```python
from build123d import *

# Parameters (mm, degrees)
BOSS_EXTRUDE1_DEPTH = 3
BOSS_EXTRUDE2_DEPTH = 3
CUT_EXTRUDE1_DEPTH  = 406.369387103
FILLET1_R           = 5
FILLET2_R           = 3.5


with BuildPart() as part:
    # Sketch1 → Boss-Extrude1 (new, symmetric)
    with BuildSketch(Plane(origin=(0, 0, 0), x_dir=(1, 0, 0), z_dir=(0, 1, 0))):
        with BuildLine():
            Line((397, -7.7), (-397, -7.7))
            ThreePointArc((-397, -7.7), (-404.7, 0), (-397, 7.7))
            Line((-397, 7.7), (397, 7.7))
            ThreePointArc((397, 7.7), (404.7, 0), (397, -7.7))
        make_face()
        with BuildLine():
            Line((397, -6.2), (-397, -6.2))
            ThreePointArc((-397, -6.2), (-403.2, 0), (-397, 6.2))
            Line((-397, 6.2), (397, 6.2))
            ThreePointArc((397, 6.2), (403.2, 0), (397, -6.2))
        make_face(mode=Mode.SUBTRACT)
    extrude(amount=BOSS_EXTRUDE1_DEPTH, both=True)

    # Sketch2 → Boss-Extrude2 (add, symmetric)
    with BuildSketch(Plane(origin=(0, 0, 0), x_dir=(1, 0, 0), z_dir=(0, 1, 0))):
        Polygon((-36.145786863, -11.5), (-36.145786863, -14.5), (-36.145786863, -22.5), (-37.645786863, -22.5), (-37.645786863, -12.137653431), (-43.807502688, -6.2), (-41.645786863, -6.2), align=None)
        Polygon((14.854213137, -14.5), (14.854213137, -11.5), (20.354213137, -6.2), (22.515928962, -6.2), (16.354213137, -12.137653431), (16.354213137, -22.5), (14.854213137, -22.5), align=None)
    extrude(amount=BOSS_EXTRUDE2_DEPTH, both=True)

    # Sketch3 → Cut-Extrude1 (cut, through all)
    with BuildSketch(Plane(origin=(0, 3, 0), x_dir=(1, 0, 0), z_dir=(0, 1, 0))):
        Polygon((-40.089183089, -7.7), (-41.645786863, -6.2), (20.354213137, -6.2), (18.797609364, -7.7), align=None)
    extrude(amount=-CUT_EXTRUDE1_DEPTH, mode=Mode.SUBTRACT)

    # Fillet1
    fillet1_edges = [part.edges().sort_by_distance(p)[0] for p in [
        (-36.145786863, 0, 11.5),
        (14.854213137, 0, 11.5),
        (-41.645786863, 0, 6.2),
        (20.354213137, 0, 6.2),
    ]]
    fillet(fillet1_edges, radius=FILLET1_R)

    # Fillet2
    fillet2_edges = [part.edges().sort_by_distance(p)[0] for p in [
        (-42.250898914, 0, 7.7),
        (-37.645786863, 0, 12.137653431),
        (20.959325189, 0, 7.7),
        (16.354213137, 0, 12.137653431),
    ]]
    fillet(fillet2_edges, radius=FILLET2_R)


solid = part.part
```
Verification items for the finished model (mm, model axes). Round coordinates to 2 decimals unless told otherwise and drop trailing zeros. Write each loop counter-clockwise with the first axis right and the second up, starting at its lowest first coordinate (ties: lowest second). Pieces come first, ordered by that corner, then holes.
1. Section check B-B on x = -107. Enter the section's corners in (y, z), plus the area to 3 significant figures.
2. Gauge pin test, flat ends, axial feed: P1, Ø1.8, axis at y = 0.5, z = 19.5, coming from the +X side; P2, Ø1, axis at y = -0.5, z = 0.5, coming from the -X side; P3, Ø1.8, axis at x = 94, y = 1.5, coming from the +Z side; P4, Ø3, axis at y = 0, z = 17, coming from the -X side. Record the tip position at first contact, or that the pin passes through.
3. Section check C-C on y = 0.5. Enter the section's corners in (x, z).
4. Scan lines: L1, parallel to Z at x = 110, y = 2.5; L2, parallel to X at y = 2.5, z = 16; L3, parallel to X at y = -1, z = 0. Record each from-to range of solid material in increasing order.
5. Section check A-A on z = 0. Enter the section's corners in (x, y), plus the area to 3 significant figures.
Answer:
1. outline: (-3, -7.7) - (3, -7.7) - (3, -6.2) - (-3, -6.2) - close; (-3, 6.2) - (3, 6.2) - (3, 7.7) - (-3, 7.7) - close
1. area: 18.0 mm2
2. P1: stops at x = 16.35
2. P2: stops at x = -404.7
2. P3: stops at z = 7.7
2. P4: stops at x = -37.65
3. outline: (-397, -7.7) - (397, -7.7) arc R7.7 ccw to (397, 7.7) - (22.37, 7.7) arc R3.5 cw to (19.94, 8.68) - (17.43, 11.11) arc R3.5 cw to (16.35, 13.63) - (16.35, 22.5) - (14.85, 22.5) - (14.85, 13.63) arc R5 ccw to (16.38, 10.03) - (18.9, 7.6) arc R5 ccw to (22.37, 6.2) - (397, 6.2) arc R6.2 cw to (397, -6.2) - (-397, -6.2) arc R6.2 cw to (-397, 6.2) - (-43.66, 6.2) arc R5 ccw to (-40.19, 7.6) - (-37.68, 10.03) arc R5 ccw to (-36.15, 13.63) - (-36.15, 22.5) - (-37.65, 22.5) - (-37.65, 13.63) arc R3.5 cw to (-38.72, 11.11) - (-41.23, 8.68) arc R3.5 cw to (-43.66, 7.7) - (-397, 7.7) arc R7.7 ccw to start
4. L1: z = -7.7 to -6.2, 6.2 to 7.7
4. L2: x = -37.65 to -36.15, 14.85 to 16.35
4. L3: x = -404.7 to -403.2, 403.2 to 404.7
5. outline: (-404.7, -3) - (-403.2, -3) - (-403.2, 3) - (-404.7, 3) - close; (403.2, -3) - (404.7, -3) - (404.7, 3) - (403.2, 3) - close
5. area: 18.0 mm2
